Verification items for the finished model (mm, model axes). Round coordinates to 2 decimals unless told otherwise and drop trailing zeros. Loops run counter-clockwise (first coordinate to the right, second up) from the corner with the lowest first, then second, coordinate; pieces in that order, holes last. Notation, with made-up numbers: M 72,49 L 101,49 A18 cw 101,84 Z; hole C 53.25,-38 d1. An arc over 180 degrees is marked long. Answer as CSV lines item,"result".
```python
from build123d import *

# Parameters (mm, degrees)
SKETCH1_R            = 38.1
BOSS_EXTRUDE1_DEPTH  = 1.5875
M4_CLEARANCE_HOLE1_D = 4.5
SKETCH4_R            = 3.3782
CUT_EXTRUDE1_DEPTH   = 4.175


with BuildPart() as part:
    # Sketch1 → Boss-Extrude1 (new body, symmetric)
    with BuildSketch(Plane(origin=(0, 0, 0), x_dir=(1, 0, 0), z_dir=(0, 1, 0))):
        Circle(SKETCH1_R)
    extrude(amount=BOSS_EXTRUDE1_DEPTH, both=True)

    # M4 Clearance Hole1 (through all)
    with Locations(Plane(origin=(0, -1.5875, 0), x_dir=(-1, 0, 0), z_dir=(0, -1, 0))):
        with Locations((-18, 0), (18, 0)):
            Hole(M4_CLEARANCE_HOLE1_D / 2)

    # Sketch4 → Cut-Extrude1 (cut, through all)
    with BuildSketch(Plane.XZ.offset(1.5875)):
        Circle(SKETCH4_R)
    extrude(amount=-CUT_EXTRUDE1_DEPTH, mode=Mode.SUBTRACT)


solid = part.part
```
1) Section check D-D (z = -25). Record the cut outline in (x, y), plus the area to 3 significant figures.
Here are the results:
outline,"M -28.75,-1.59 L 28.75,-1.59 L 28.75,1.59 L -28.75,1.59 Z"
area,"183 mm^2"
2) Draft check along Z on faces 1 (the flat face through (8, 1.588, -1)), 2 (the cylindrical face through (-15.854, 0.022, -0.676)), 3 (the cylindrical face through (-30.235, 0.022, 23.183)). Enter one of: +Z half, -Z half, draft (parallel to the pull), parting line (faces both ways), or undercut.
Here are the results:
face 1,"draft"
face 2,"undercut"
face 3,"parting line"
3) Material ranges on probe 1 along Z at (x, y) = (0, 0.75); probe 2 along Z at (x, y) = (1.5, 1.45); probe 3 along Z at (x, y) = (-20.5, 0.2), recorded low to high.
Here are the results:
probe 1,"z = -38.1 to -3.38, 3.38 to 38.1"
probe 2,"z = -38.07 to -3.03, 3.03 to 38.07"
probe 3,"z = -32.11 to 32.11"
4) Go/stop test with flat-tipped pins: pin 1 (11 mm diameter, centred on x = 0, z = 0, fed in from -Y); pin 2 (1 mm diameter, centred on x = 21, y = 0, fed in from +Z); pin 3 (1.5 mm diameter, centred on x = -2, y = 0, fed in from +Z). Record where each tip stops, or that it passes through.
Here are the results:
pin 1,"stops at y = -1.59"
pin 2,"stops at z = 32.11"
pin 3,"stops at z = 38.08"
5) Section check C-C (x = 18). Record the cut outline in (y, z).
Here are the results:
outline,"M -1.59,-33.58 L 1.59,-33.58 L 1.59,-2.25 L -1.59,-2.25 Z; M -1.59,2.25 L 1.59,2.25 L 1.59,33.58 L -1.59,33.58 Z"
6) Section check A-A (x = 0). Record the cut outline in (y, z).
Here are the results:
outline,"M -1.59,-38.1 L 1.59,-38.1 L 1.59,-3.38 L -1.59,-3.38 Z; M -1.59,3.38 L 1.59,3.38 L 1.59,38.1 L -1.59,38.1 Z"
7) Section check B-B (y = 0.85). Record the cut outline in (x, z).
Here are the results:
outline,"C 0,0 d76.2; hole C -18,0 d4.5; hole C 0,0 d6.76; hole C 18,0 d4.5"
